The drawing under review shows one solid part. Ordinate dimensions are in mm from its lowest x, y, z. Give positions to 0.01 mm unless a question says otherwise; leave off trailing zeros. Loops run counter-clockwise (first coordinate to the right, second up) from the corner with the lowest first, then second, coordinate; pieces in that order, holes last. Notation, with made-up numbers: (3.25, 63) -> (23.25, 63) arc R28 cw to (23.25, 94) -> close; hole circle Ø4 at (20, 65.5). An arc over 180 degrees is marked (long way). Answer in a Markdown table with one row per item. Add a question column.
(1) Consider section D-D on z = 93.5. Write out the cut boundary in (x, y).
(2) Consider section A-A on y = 1.3. Write out the cut boundary in (x, z).
(3) Consider section B-B on z = 50. Write out the cut boundary in (x, y).
(4) Consider section C-C on x = 26. Write out the cut boundary in (y, z), then the cut area to 3 significant figures.
(5) For line 1 (Z direction, x = 97.35, y = 2.2); line 2 (Z direction, x = 87.4, y = 2.15); line 3 (Z direction, x = 88.5, y = 1.45), list the stretches that pass through material, from the lowest coordinate up.
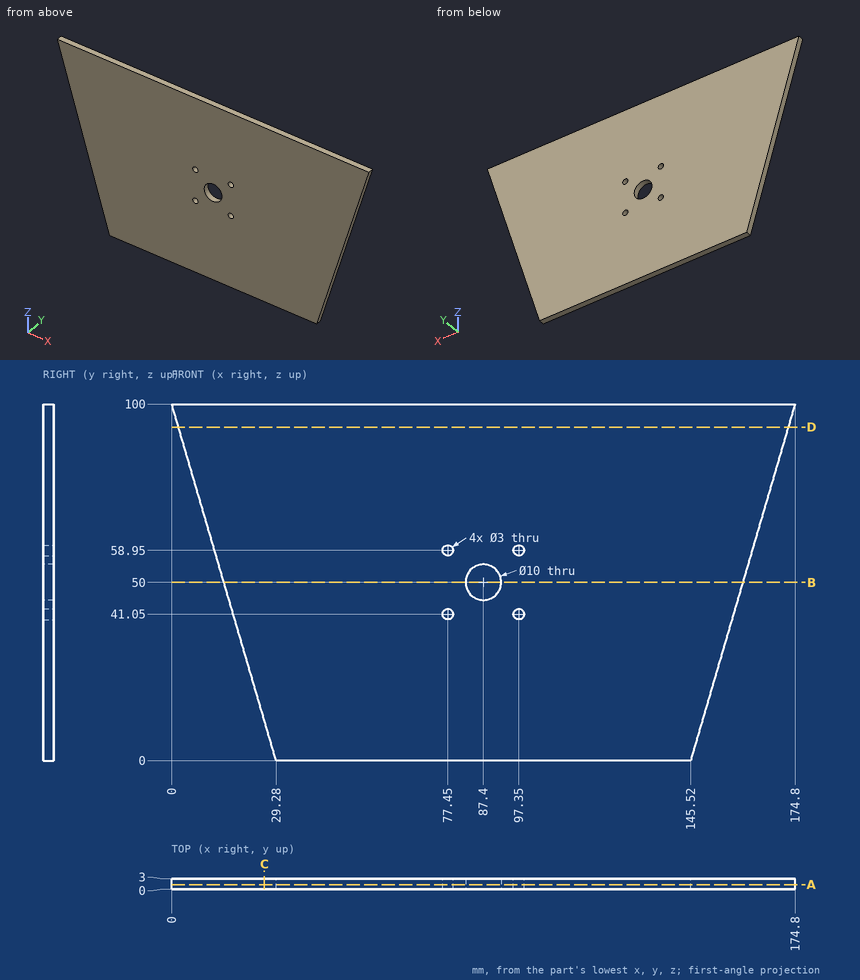
Values follow:
| question | item | result |
|---|---|---|
| 1 | outline | (1.9, 0) -> (172.9, 0) -> (172.9, 3) -> (1.9, 3) -> close |
| 2 | outline | (0, 100) -> (29.28, 0) -> (145.52, 0) -> (174.8, 100) -> close; hole circle Ø3 at (77.45, 41.05); hole circle Ø3 at (77.45, 58.95); hole circle Ø10 at (87.4, 50); hole circle Ø3 at (97.35, 41.05); hole circle Ø3 at (97.35, 58.95) |
| 3 | outline | (14.64, 0) -> (82.4, 0) -> (82.4, 3) -> (14.64, 3) -> close; (92.4, 0) -> (160.16, 0) -> (160.16, 3) -> (92.4, 3) -> close |
| 4 | outline | (0, 11.2) -> (3, 11.2) -> (3, 100) -> (0, 100) -> close |
| 4 | area | 266 mm2 |
| 5 | line 1 | 0 to 39.55, 42.55 to 57.45, 60.45 to 100 |
| 5 | line 2 | 0 to 45, 55 to 100 |
| 5 | line 3 | 0 to 45.12, 54.88 to 100 |
